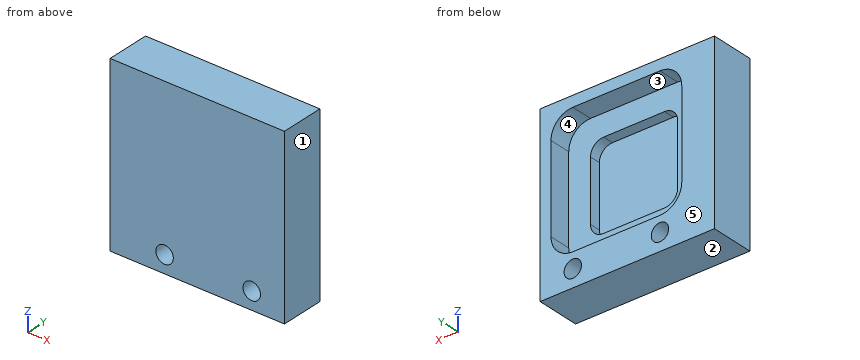
from build123d import *

# Parameters (mm, degrees)
F0_W     = 80
F0_H     = 80
F1_DEPTH = 20
F3_DEPTH = 15
F5_DEPTH = 10
F6_R     = 4
F7_DEPTH = 25


with BuildPart() as f1:
    # F0 (on Front) → F1 (new body)
    with BuildSketch(Plane.XZ):
        Rectangle(F0_W, F0_H)
    extrude(amount=F1_DEPTH)

    # F2 (on face) → F3 (cut)
    with BuildSketch(Plane(origin=(0, 0, 0), x_dir=(-1, 0, 0), z_dir=(0, 1, 0))):
        with BuildLine():
            ThreePointArc((-19, 25), (-23.242641, 23.242641), (-25, 19))
            Line((-25, 19), (-25, -9))
            ThreePointArc((-25, -9), (-23.242641, -13.242641), (-19, -15))
            Line((-19, -15), (9, -15))
            ThreePointArc((9, -15), (13.242641, -13.242641), (15, -9))
            Line((15, -9), (15, 19))
            ThreePointArc((15, 19), (13.242641, 23.242641), (9, 25))
            Line((9, 25), (-19, 25))
        make_face()
    extrude(amount=-F3_DEPTH, mode=Mode.SUBTRACT)

    # F4 (on face) → F5 (cut)
    with BuildSketch(Plane(origin=(0, 0, 0), x_dir=(-1, 0, 0), z_dir=(0, 1, 0))):
        with BuildLine():
            Line((-35, 25), (-35, -15))
            ThreePointArc((-35, -15), (-32.071068, -22.071068), (-25, -25))
            Line((-25, -25), (15, -25))
            ThreePointArc((15, -25), (22.071068, -22.071068), (25, -15))
            Line((25, -15), (25, 25))
            ThreePointArc((25, 25), (22.071068, 32.071068), (15, 35))
            Line((15, 35), (-25, 35))
            ThreePointArc((-25, 35), (-32.071068, 32.071068), (-35, 25))
        make_face()
    extrude(amount=-F5_DEPTH, mode=Mode.SUBTRACT)

    # F6 (on face) → F7 (cut)
    with BuildSketch(Plane(origin=(0, 0, 0), x_dir=(-1, 0, 0), z_dir=(0, 1, 0))):
        with Locations((-25, -32)):
            Circle(F6_R)
        with Locations((15, -32)):
            Circle(F6_R)
    extrude(amount=-F7_DEPTH, mode=Mode.SUBTRACT)


solid = f1.part
Work out the finished part from the listing and answer in its coordinate system (mm). Face numbers are marked on the shaded views. A direction names the side the tool comes from. Round coordinates to 2 decimals unless told otherwise and drop trailing zeros. Loops run counter-clockwise (first coordinate to the right, second up) from the corner with the lowest first, then second, coordinate; pieces in that order, holes last. Notation, with made-up numbers: M 6,22.5 L 35,22.5 A35 cw 35,54.5 Z; hole C 17,21 d11. An arc over 180 degrees is marked long. One line per question, with ' | ' between items. Start each with the question number.
(1) A tool of negligible diameter and unlimited length cuts with its end or side. For the marked faces 4 and 5, from which of +Z, -Z, +X, -X, +Y, -Y can it reach the whole face along a straight path? Write none if from no direction.
(2) For a pull along Z with two mould halves and no side action, classify the marked faces 1, 2 and 3 as released by +Z, released by -Z, zero draft, split by the parting line, or undercut.
(3) Find the intervals of material crossed by line 1 (Z direction, x = 25, y = -4.25); line 2 (X direction, y = -5.5, z = 17.5); line 3 (X direction, y = -12, z = 6.5), in increasing order.
(4) A cutting plane is placed at A-A on z = -32. Write down the section's boundary in (x, y), plus the area to 3 significant figures.
(5) A cutting plane is placed at D-D on y = -18. Write down the section's boundary in (x, z), plus the area to 3 significant figures.
(6) A cutting plane is placed at B-B on y = -7.75. Write down the section's boundary in (x, z), plus the area to 3 significant figures.
(7) A flat-ended cylindrical pin translates along its axis: pin 1 Ø7 at (x, z) = (-15, -32) entering from -Y. Find the tip coordinate at first contact, or state that the pin passes through.
(8) A cutting plane is placed at C-C on z = 33. Write down the section's boundary in (x, y), plus the area to 3 significant figures.
Geometry check:
1) face 4: +Y | face 5: +Z, -Z, +X, -X, +Y
2) face 1: zero draft | face 2: released by -Z | face 3: undercut
3) line 1: z = -40 to -36, -28 to -25, 35 to 40 | line 2: x = -40 to -25, 35 to 40 | line 3: x = -40 to -15, 25 to 40
4) outline: M -40,-20 L -19,-20 L -19,0 L -40,0 Z; M -11,-20 L 21,-20 L 21,0 L -11,0 Z; M 29,-20 L 40,-20 L 40,0 L 29,0 Z | area: 1,280 mm²
5) outline: M -40,-40 L 40,-40 L 40,40 L -40,40 Z; hole C -15,-32 d8; hole C 25,-32 d8 | area: 6,300 mm²
6) outline: M -40,-40 L 40,-40 L 40,40 L -40,40 Z; hole M -25,-15 A10 ccw -15,-25 L 25,-25 A10 ccw 35,-15 L 35,25 A10 ccw 25,35 L -15,35 A10 ccw -25,25 Z; hole C -15,-32 d8; hole C 25,-32 d8 | area: 2,790 mm²
7) pin 1: passes through
8) outline: M -40,-20 L 40,-20 L 40,0 L 31,0 L 31,-10 L -21,-10 L -21,0 L -40,0 Z | area: 1,080 mm²
